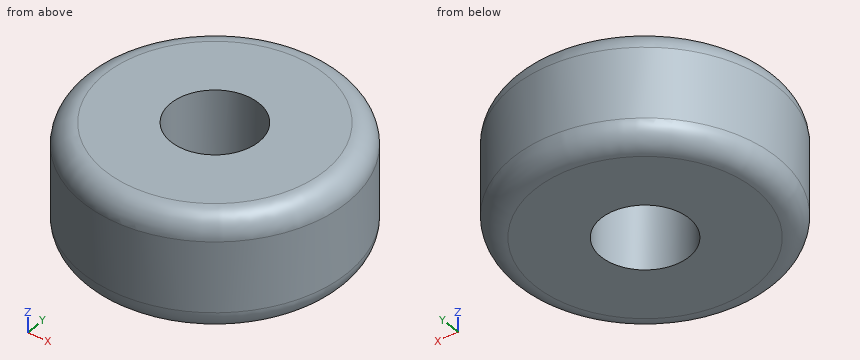
```python
from build123d import *

# Parameters (mm, degrees)
ESQUISSE1_R             = 12
BOSS_EXTRU_1_DEPTH      = 10.4
CONG_1_R                = 2
CONG_2_R                = 2
ESQUISSE2_R             = 4
ENL_V_MAT_EXTRU_1_DEPTH = 10.4


with BuildPart() as part:
    # Esquisse1 → Boss.-Extru.1 (new body)
    with BuildSketch(Plane.XY):
        Circle(ESQUISSE1_R)
    extrude(amount=BOSS_EXTRU_1_DEPTH)

    # Congé1
    cong_1_edges = [part.edges().sort_by_distance(p)[0] for p in [
        (-12, 0, 10.4),
    ]]
    fillet(cong_1_edges, radius=CONG_1_R)

    # Congé2
    cong_2_edges = [part.edges().sort_by_distance(p)[0] for p in [
        (-12, 0, 0),
    ]]
    fillet(cong_2_edges, radius=CONG_2_R)

    # Esquisse2 → Enlèv. mat.-Extru.1 (cut)
    with BuildSketch(Plane.XY):
        Circle(ESQUISSE2_R)
    extrude(amount=ENL_V_MAT_EXTRU_1_DEPTH, mode=Mode.SUBTRACT)


solid = part.part
```
Geometry: final body of the model. Coordinates: model frame, mm. Give positions to 0.01 mm unless a question says otherwise; leave off trailing zeros. Loops run counter-clockwise (first coordinate to the right, second up) from the corner with the lowest first, then second, coordinate; pieces in that order, holes last. Notation, with made-up numbers: (31, -13.75) -> (39, -13.75) arc R20 cw to (39, -3.75) -> close; hole circle Ø2 at (-19, 16.25). An arc over 180 degrees is marked (long way). Return JSON: item names as keys, results as strings.
Item 1: Section C-C, the plane z = 3.5. Output: boundary loops of the cut face in (x, y).
Filled in:
{"outline": "circle Ø24 at (0, 0); hole circle Ø8 at (0, 0)"}
Item 2: Section A-A, the plane y = 0. Output: boundary loops of the cut face in (x, z), plus the area to 3 significant figures.
Filled in:
{"outline": "(-12, 2) arc R2 ccw to (-10, 0) -> (-4, 0) -> (-4, 10.4) -> (-10, 10.4) arc R2 ccw to (-12, 8.4) -> close; (4, 0) -> (10, 0) arc R2 ccw to (12, 2) -> (12, 8.4) arc R2 ccw to (10, 10.4) -> (4, 10.4) -> close", "area": "163 mm^2"}
Item 3: Line query: line 1 (Y direction, x = 0, z = 3.75); line 2 (X direction, y = 2.25, z = 6); line 3 (Y direction, x = 3.25, z = 1). Output: solid intervals per line, ascending.
Filled in:
{"line 1": "-12 to -4, 4 to 12", "line 2": "-11.79 to -3.31, 3.31 to 11.79", "line 3": "-11.27 to -2.33, 2.33 to 11.27"}
Item 4: Pin query (flat end, axial travel): P1, Ø9, axis at x = 0, y = 0, coming from the -Z side; P2, Ø1, axis at y = -2.5, z = 7.5, coming from the -X side; P3, Ø1.5, axis at x = 9, z = 4, coming from the -Y side; P4, Ø4, axis at y = 3, z = 7, coming from the -X side. Return the tip coordinate at first contact, or that it passes through.
Filled in:
{"P1": "z = 0", "P2": "x = -11.83", "P3": "y = -8.71", "P4": "x = -11.96"}
